```python
from build123d import *

# Parameters (mm, degrees)
F0_R     = 3.175
F1_DEPTH = 3.048


with BuildPart() as f1:
    # F0 (on Front) → F1 (new body)
    with BuildSketch(Plane.XZ):
        with BuildLine():
            ThreePointArc((3.175, 114.3), (-2.245064, 116.545064), (0, 111.125))
            ThreePointArc((0, 111.125), (2.245064, 112.054936), (3.175, 114.3))
        make_face()
        with BuildLine():
            ThreePointArc((0, 104.775), (6.735192, 107.564808), (9.525, 114.3))
            ThreePointArc((9.525, 114.3), (9.506305, 114.896482), (9.450293, 115.490622))
            ThreePointArc((9.450293, 115.490622), (-0.596482, 123.806305), (-9.525, 114.3))
            ThreePointArc((-9.525, 114.3), (-6.735192, 107.564808), (0, 104.775))
        make_face()
        with BuildLine():
            ThreePointArc((3.175, 114.3), (2.245064, 112.054936), (0, 111.125))
            ThreePointArc((0, 111.125), (-2.245064, 116.545064), (3.175, 114.3))
        make_face(mode=Mode.SUBTRACT)
        with BuildLine():
            ThreePointArc((9.450293, 115.490622), (9.506305, 114.896482), (9.525, 114.3))
            ThreePointArc((9.525, 114.3), (6.735192, 107.564808), (0, 104.775))
            Line((0, 104.775), (0, 100.0252))
            Line((0, 100.0252), (0, 79.375))
            ThreePointArc((0, 79.375), (10.491283, 75.414219), (15.747457, 65.508289))
            Line((15.747457, 65.508289), (9.450293, 115.490622))
        make_face()
        with BuildLine():
            Line((0, 100.0252), (0, 104.775))
            ThreePointArc((0, 104.775), (-6.735192, 107.564808), (-9.525, 114.3))
            Line((-9.525, 114.3), (-15.747457, 65.508289))
            ThreePointArc((-15.747457, 65.508289), (-10.491283, 75.414219), (0, 79.375))
            Line((0, 79.375), (0, 100.0252))
        make_face()
        with Locations((-3.175, 100.0252)):
            Circle(F0_R, mode=Mode.SUBTRACT)
        with BuildLine():
            ThreePointArc((15.875, 63.5), (15.843082, 64.506168), (15.747457, 65.508289))
            ThreePointArc((15.747457, 65.508289), (10.491283, 75.414219), (0, 79.375))
            Line((0, 79.375), (0, 66.675))
            ThreePointArc((0, 66.675), (2.245064, 65.745064), (3.175, 63.5))
            ThreePointArc((3.175, 63.5), (2.245064, 61.254936), (0, 60.325))
            Line((0, 60.325), (0, 47.625))
            ThreePointArc((0, 47.625), (10.491283, 51.585781), (15.747457, 61.491711))
            ThreePointArc((15.747457, 61.491711), (15.843082, 62.493832), (15.875, 63.5))
        make_face()
        with BuildLine():
            ThreePointArc((0, 79.375), (-10.491283, 75.414219), (-15.747457, 65.508289))
            ThreePointArc((-15.747457, 65.508289), (-15.875, 63.5), (-15.747457, 61.491711))
            ThreePointArc((-15.747457, 61.491711), (-10.491283, 51.585781), (0, 47.625))
            Line((0, 47.625), (0, 60.325))
            ThreePointArc((0, 60.325), (-3.175, 63.5), (0, 66.675))
            Line((0, 66.675), (0, 79.375))
        make_face()
        with BuildLine():
            ThreePointArc((0, 47.625), (-10.491283, 51.585781), (-15.747457, 61.491711))
            Line((-15.747457, 61.491711), (-9.525, 0))
            ThreePointArc((-9.525, 0), (-6.735192, 6.735192), (0, 9.525))
            Line((0, 9.525), (0, 47.625))
        make_face()
        with BuildLine():
            Line((9.959056, 16.103534), (15.747457, 61.491711))
            ThreePointArc((15.747457, 61.491711), (10.491283, 51.585781), (0, 47.625))
            Line((0, 47.625), (0, 9.525))
            ThreePointArc((0, 9.525), (6.735192, 6.735192), (9.525, 0))
            Line((9.525, 0), (36.5125, 0))
            ThreePointArc((36.5125, 0), (38.93809, 5.711633), (44.732405, 7.932475))
            Line((44.732405, 7.932475), (16.032115, 8.954238))
            ThreePointArc((16.032115, 8.954238), (11.418441, 11.189161), (9.959056, 16.103534))
        make_face()
        with BuildLine():
            ThreePointArc((0, 9.525), (-6.735192, 6.735192), (-9.525, 0))
            ThreePointArc((-9.525, 0), (-6.735192, -6.735192), (0, -9.525))
            Line((0, -9.525), (0.677344, -9.500886))
            ThreePointArc((0.677344, -9.500886), (6.970557, -6.491299), (9.525, 0))
            Line((9.525, 0), (3.175, 0))
            ThreePointArc((3.175, 0), (-2.245064, -2.245064), (0, 3.175))
            Line((0, 3.175), (0, 9.525))
        make_face()
        with BuildLine():
            Line((0.677344, -9.500886), (0, -9.525))
            ThreePointArc((0, -9.525), (0.338886, -9.51897), (0.677344, -9.500886))
        make_face()
        with BuildLine():
            Line((36.5125, 0), (9.525, 0))
            ThreePointArc((9.525, 0), (6.970557, -6.491299), (0.677344, -9.500886))
            Line((0.677344, -9.500886), (44.732405, -7.932475))
            ThreePointArc((44.732405, -7.932475), (38.93809, -5.711633), (36.5125, 0))
        make_face()
        with BuildLine():
            ThreePointArc((47.625, 0), (44.45, 3.175), (41.275, 0))
            ThreePointArc((41.275, 0), (44.45, -3.175), (47.625, 0))
        make_face()
        with BuildLine():
            ThreePointArc((52.3875, 0), (50.161633, 5.51191), (44.732405, 7.932475))
            ThreePointArc((44.732405, 7.932475), (38.93809, 5.711633), (36.5125, 0))
            ThreePointArc((36.5125, 0), (38.93809, -5.711633), (44.732405, -7.932475))
            ThreePointArc((44.732405, -7.932475), (50.161633, -5.51191), (52.3875, 0))
        make_face()
        with BuildLine():
            ThreePointArc((47.625, 0), (44.45, -3.175), (41.275, 0))
            ThreePointArc((41.275, 0), (44.45, 3.175), (47.625, 0))
        make_face(mode=Mode.SUBTRACT)
    extrude(amount=F1_DEPTH)


solid = f1.part
```
Design review of the part built by this model. Coordinates are the model's own, in mm. A direction names the side the tool comes from. Coordinates: 2 decimals unless noted, no trailing zeros. Write each loop counter-clockwise with the first axis right and the second up, starting at its lowest first coordinate (ties: lowest second). Pieces come first, ordered by that corner, then holes.
1) Add section A-A (x = 14.5). Write out the cut boundary in (y, z), plus the area to 3 significant figures.
2) Machinability: for faces 4 (the flat face through (0, -2, 6)), 5 (the flat face through (12.813, -1.503, 38.48)), 6 (the flat face through (-12.68, -1.5, 31.18)), which of the approach directions +Z, -Z, +X, -X, +Y, -Y give a long, thin tool a straight path to every point of the face, cutting with its end or side? Answer none if there is none.
3) To check wall thickness, follow L1, parallel to X at y = -2.25, z = 0.5; L2, parallel to X at y = -1.7, z = 114.3 (3 decimals); L3, parallel to Z at x = 44.45, y = -1.2 (3 decimals). State the ranges of each line that lie inside material, in increasing order.
4) Add section D-D (z = 40). Write out the cut boundary in (x, y), plus the area to 3 significant figures.
5) Add section C-C (y = -2.45). State how many separate pieces and enclosed holes the cut face has, plus the area to 3 significant figures.
6) Add section B-B (z = 5.5). Write out the cut boundary in (x, y).
7) Insertion check: pin 1 (1.5 mm diameter, centred on x = 29, y = -1, fed in from -Z); pin 2 (0.9 mm diameter, centred on y = -1.5, z = 7.5, fed in from +X). Each pin has a flat end and moves straight along its axis. Give the tip position at first contact, or say it passes through.
8) Mouldability with a two-part tool opening along Z and no side actions: class faces 1 (the cylindrical face through (-6.81, -1.5, -6.66)), 2 (the cylindrical face through (-2.17, -1.5, -2.32)), 3 (the flat face through (3, 0, 43)) as +Z half, -Z half, draft (parallel to the pull), parting line (faces both ways), or undercut.
Check result:
1. outline: (-3.05, -9.01) - (0, -9.01) - (0, 9.2) - (-3.05, 9.2) - close; (-3.05, 51.71) - (0, 51.71) - (0, 75.41) - (-3.05, 75.41) - close
1. area: 128 mm2
2. face 4: +Y, -Y
2. face 5: +X, +Y, -Y
2. face 6: -Z, -X, +Y, -Y
3. L1: x = -9.58 to -3.14, 9.51 to 41.31, 47.59 to 52.37
3. L2: x = -9.525 to -3.175, 3.175 to 9.6
3. L3: z = -7.943 to -3.175, 3.175 to 7.943
4. outline: (-13.57, -3.05) - (13.01, -3.05) - (13.01, 0) - (-13.57, 0) - close
4. area: 81.0 mm2
5. separate pieces: 1
5. enclosed holes: 5
5. area: 3,660 mm2
6. outline: (-10.08, -3.05) - (0, -3.05) - (0, 0) - (-10.08, 0) - close; (7.78, -3.05) - (50.17, -3.05) - (50.17, 0) - (7.78, 0) - close
7. pin 1: stops at z = -8.52
7. pin 2: stops at x = 48.1
8. face 1: -Z half
8. face 2: undercut
8. face 3: draft
